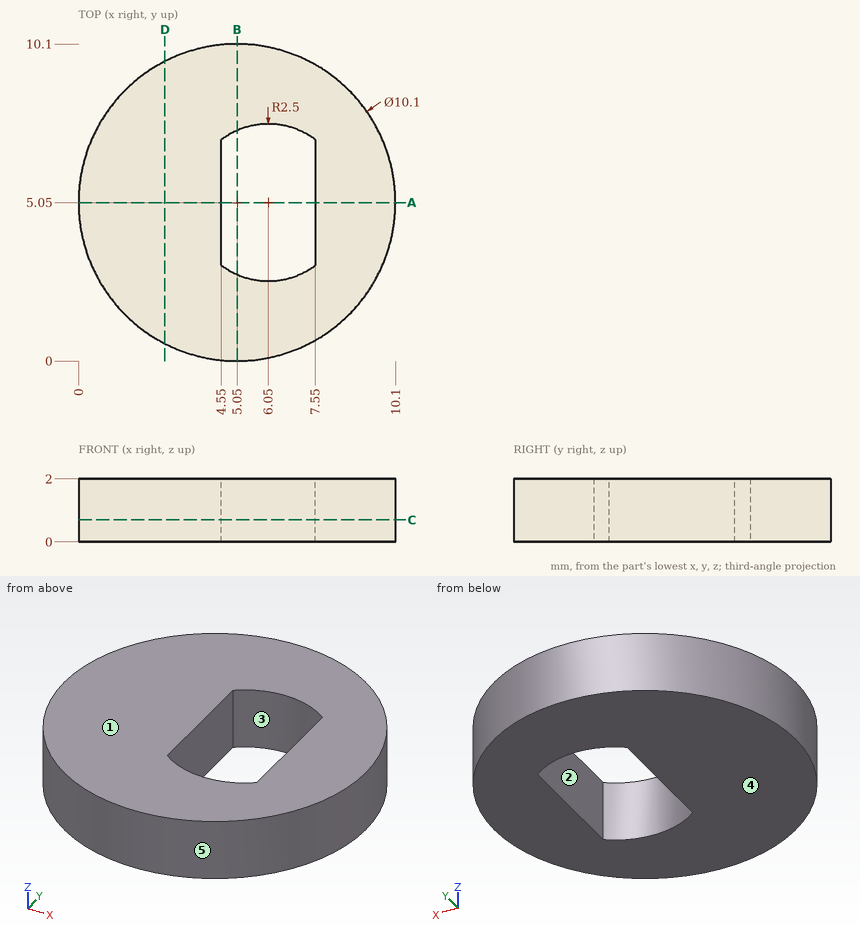
Answer from the drawing. Dimensions are ordinates in mm from the lowest x, y and z of the part. A direction names the side the tool comes from. Round coordinates to 2 decimals unless told otherwise and drop trailing zeros. Order: outer loops, then holes, each group sorted by start corner. A loop starts at its lowest first (then second) coordinate and runs counter-clockwise, first axis right, second up.
1) The mould has two halves that part along X. Classify the marked faces 3, 4 and 5: released by +X, released by -X, zero draft, split by the parting line, or undercut.
2) The part is cut by section D-D on x = 2.75. Write down the section's boundary in (y, z), plus the area to 3 significant figures.
3) The part is cut by section B-B on x = 5.05. Write down the section's boundary in (y, z).
4) The part is cut by section A-A on y = 5.05. Write down the section's boundary in (x, z), plus the area to 3 significant figures.
5) For the marked faces 1 and 2, determine the directions among +Z, -Z, +X, -X, +Y, -Y from which every point of the face is accessible in a straight line to the end or side of a thin tool.
6) A flat-ended cylindrical pin translates along its axis: pin 1 (0.6 mm diameter, centred on y = 4.5, z = 1, fed in from +X). Find the tip coordinate at first contact, or state that the pin passes through.
7) Straight lines are drawn through the part: L1, parallel to Y at x = 7, z = 1.45; L2, parallel to Y at x = 6.5, z = 0.9; L3, parallel to X at y = 3.25, z = 1.45. For each, find the intervals that lie inside material, in ascending order.
8) The part is cut by section C-C on z = 0.7. Write down the section's boundary in (x, y), plus the area to 3 significant figures.
Resolved:
1. face 3: undercut
1. face 4: zero draft
1. face 5: split by the parting line
2. outline: (0.55, 0) - (9.55, 0) - (9.55, 2) - (0.55, 2) - close
2. area: 18.0 mm2
3. outline: (0, 0) - (2.76, 0) - (2.76, 2) - (0, 2) - close; (7.34, 0) - (10.1, 0) - (10.1, 2) - (7.34, 2) - close
4. outline: (0, 0) - (4.55, 0) - (4.55, 2) - (0, 2) - close; (7.55, 0) - (10.1, 0) - (10.1, 2) - (7.55, 2) - close
4. area: 14.2 mm2
5. face 1: +Z, +X, -X, +Y, -Y
5. face 2: +Z, -Z
6. pin 1: stops at x = 10.09
7. L1: y = 0.39 to 2.74, 7.36 to 9.71
7. L2: y = 0.21 to 2.59, 7.51 to 9.89
7. L3: x = 0.33 to 4.55, 7.55 to 9.77
8. outline: circle Ø10.1 at (5.05, 5.05); hole (4.55, 3.05) arc R2.5 ccw to (7.55, 3.05) - (7.55, 7.05) arc R2.5 ccw to (4.55, 7.05) - close
8. area: 66.1 mm2
